Source: CAD feature listing. Evaluate the final solid. Frame: model axes, mm. Face numbers are marked on the shaded views. Give positions to 0.01 mm unless a question says otherwise; leave off trailing zeros. Loops run counter-clockwise (first coordinate to the right, second up) from the corner with the lowest first, then second, coordinate; pieces in that order, holes last. Notation, with made-up numbers: (-21.75, 60) -> (-14.75, 60) arc R17 cw to (-14.75, 93) -> close; hole circle Ø6 at (35, -12.5). An arc over 180 degrees is marked (long way). Return JSON: item names as keys, results as strings. Group by question number.
(1) Ray query, line 1 (Y direction, x = 35, z = 94); line 2 (X direction, y = 21.25, z = 50.8); line 3 (X direction, y = 16, z = 88). Return the intervals inside material, ascending. Write a range as from..to.
(2) Pin query (flat end, axial travel): pin 1 (6.5 mm diameter, centred on y = 9.5, z = 32.5, fed in from -X); pin 2 (10 mm diameter, centred on x = 27.5, y = 12.5, fed in from +Z); pin 3 (17 mm diameter, centred on x = 25.4, z = 50.8, fed in from +Y). Return the tip coordinate at first contact, or that it passes through.
(3) Cut plane C-C on z = 50.8. Return loops of the section in (x, y).
(4) Cut plane B-B on y = 13.25. Return loops of the section in (x, z).
(5) Cut plane D-D on x = 9.5. Return loops of the section in (y, z), then the cut area to 3 significant figures.
(6) Draft query along Y for the marked faces 1, 2, 3 and 4. Return one class per face: released by +Y, released by -Y, zero draft, split by the parting line, or undercut.
(7) Cut plane A-A on x = 25.4. Return loops of the section in (y, z), then the cut area to 3 significant figures.
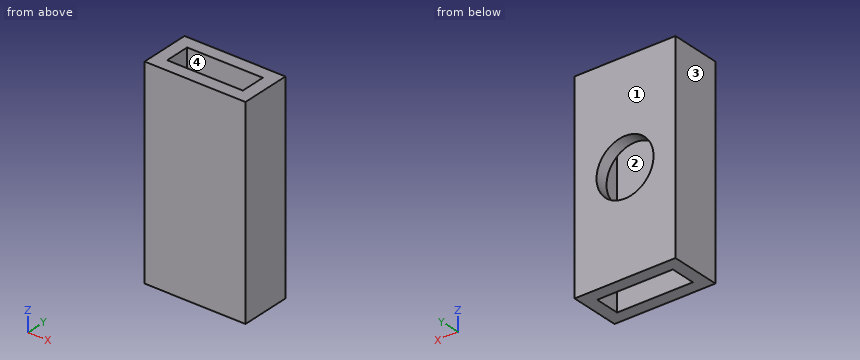
```python
from build123d import *

# Parameters (mm, degrees)
SKETCH1_W           = 50.8
SKETCH1_H           = 25.4
BOSS_EXTRUDE1_DEPTH = 101.6
SKETCH2_W           = 38.1
SKETCH2_H           = 12.7
CUT_EXTRUDE1_DEPTH  = 117.397422652
CUT_EXTRUDE3_REACH  = 118.397
SKETCH5_R           = 14.351


with BuildPart() as part:
    # Sketch1 → Boss-Extrude1 (new body)
    with BuildSketch(Plane.XY):
        with Locations((25.4, 12.7)):
            Rectangle(SKETCH1_W, SKETCH1_H)
    extrude(amount=BOSS_EXTRUDE1_DEPTH)

    # Sketch2 → Cut-Extrude1 (cut, through all)
    with BuildSketch(Plane.XY.offset(101.6)):
        with Locations((25.4, 12.7)):
            Rectangle(SKETCH2_W, SKETCH2_H)
    extrude(amount=-CUT_EXTRUDE1_DEPTH, mode=Mode.SUBTRACT)

    # Sketch5 → Cut-Extrude3 (cut, up to next)
    with BuildSketch(Plane(origin=(0, 25.4, 0), x_dir=(1, 0, 0), z_dir=(0, 1, 0)), mode=Mode.PRIVATE) as cut_extrude3_sk1:
        with Locations(Location((25.4, -50.8, 0), (0, 0, 270))):
            Circle(SKETCH5_R)
    cut_extrude3_tool1 = extrude(cut_extrude3_sk1.sketch, amount=-CUT_EXTRUDE3_REACH, mode=Mode.PRIVATE) & part.part
    add(cut_extrude3_tool1.solids().sort_by_distance((25.4, 25.4, 50.8))[0], mode=Mode.SUBTRACT)


solid = part.part
```
Answers:
{
 "1": {"line 1": "0..6.35, 19.05..25.4", "line 2": "0..11.05, 39.75..50.8", "line 3": "0..6.35, 44.45..50.8"},
 "2": {"pin 1": "x = 0", "pin 2": "through", "pin 3": "y = 6.35"},
 "3": {"outline": "(0, 0) -> (50.8, 0) -> (50.8, 25.4) -> (39.75, 25.4) -> (39.75, 19.05) -> (44.45, 19.05) -> (44.45, 6.35) -> (6.35, 6.35) -> (6.35, 19.05) -> (11.05, 19.05) -> (11.05, 25.4) -> (0, 25.4) -> close"},
 "4": {"outline": "(0, 0) -> (6.35, 0) -> (6.35, 101.6) -> (0, 101.6) -> close; (44.45, 0) -> (50.8, 0) -> (50.8, 101.6) -> (44.45, 101.6) -> close"},
 "5": {"outline": "(0, 0) -> (6.35, 0) -> (6.35, 101.6) -> (0, 101.6) -> close; (19.05, 0) -> (25.4, 0) -> (25.4, 101.6) -> (19.05, 101.6) -> close", "area": "1,290 mm²"},
 "6": {"face 1": "released by +Y", "face 2": "undercut", "face 3": "zero draft", "face 4": "undercut"},
 "7": {"outline": "(0, 0) -> (6.35, 0) -> (6.35, 101.6) -> (0, 101.6) -> close; (19.05, 0) -> (25.4, 0) -> (25.4, 36.45) -> (19.05, 36.45) -> close; (19.05, 65.15) -> (25.4, 65.15) -> (25.4, 101.6) -> (19.05, 101.6) -> close", "area": "1,110 mm²"}
}
